from build123d import *

# Parameters (mm, degrees)
SKETCH1_W                  = 650
SKETCH1_H                  = 400
BOSS_EXTRUDE1_DEPTH        = 12
FILLET1_R                  = 10
SKETCH31_R                 = 8.15
CUT_EXTRUDE3_DEPTH         = 764.311207831
LPATTERN1_COUNT            = 9
LPATTERN1_PITCH            = 50
LPATTERN2_COUNT            = 4
LPATTERN2_PITCH            = 50
LPATTERN2_COPY_1_SKETCH_R  = 8.15
LPATTERN2_COPY_1_DEPTH     = 764.311207831
LPATTERN2_COPY_2_SKETCH_R  = 8.15
LPATTERN2_COPY_2_DEPTH     = 764.311207831
LPATTERN2_COPY_3_SKETCH_R  = 8.15
LPATTERN2_COPY_3_DEPTH     = 764.311207831
LPATTERN2_COPY_4_SKETCH_R  = 8.15
LPATTERN2_COPY_4_DEPTH     = 764.311207831
LPATTERN2_COPY_5_SKETCH_R  = 8.15
LPATTERN2_COPY_5_DEPTH     = 764.311207831
LPATTERN2_COPY_6_SKETCH_R  = 8.15
LPATTERN2_COPY_6_DEPTH     = 764.311207831
LPATTERN2_COPY_7_SKETCH_R  = 8.15
LPATTERN2_COPY_7_DEPTH     = 764.311207831
LPATTERN2_COPY_8_SKETCH_R  = 8.15
LPATTERN2_COPY_8_DEPTH     = 764.311207831
LPATTERN2_COPY_9_SKETCH_R  = 8.15
LPATTERN2_COPY_9_DEPTH     = 764.311207831
LPATTERN2_COPY_10_SKETCH_R = 8.15
LPATTERN2_COPY_10_DEPTH    = 764.311207831
LPATTERN2_COPY_11_SKETCH_R = 8.15
LPATTERN2_COPY_11_DEPTH    = 764.311207831
LPATTERN2_COPY_12_SKETCH_R = 8.15
LPATTERN2_COPY_12_DEPTH    = 764.311207831
LPATTERN2_COPY_13_SKETCH_R = 8.15
LPATTERN2_COPY_13_DEPTH    = 764.311207831
LPATTERN2_COPY_14_SKETCH_R = 8.15
LPATTERN2_COPY_14_DEPTH    = 764.311207831
LPATTERN2_COPY_15_SKETCH_R = 8.15
LPATTERN2_COPY_15_DEPTH    = 764.311207831
LPATTERN2_COPY_16_SKETCH_R = 8.15
LPATTERN2_COPY_16_DEPTH    = 764.311207831
LPATTERN2_COPY_17_SKETCH_R = 8.15
LPATTERN2_COPY_17_DEPTH    = 764.311207831
LPATTERN2_COPY_18_SKETCH_R = 8.15
LPATTERN2_COPY_18_DEPTH    = 764.311207831
LPATTERN2_COPY_19_SKETCH_R = 8.15
LPATTERN2_COPY_19_DEPTH    = 764.311207831
LPATTERN2_COPY_20_SKETCH_R = 8.15
LPATTERN2_COPY_20_DEPTH    = 764.311207831
LPATTERN2_COPY_21_SKETCH_R = 8.15
LPATTERN2_COPY_21_DEPTH    = 764.311207831
LPATTERN2_COPY_22_SKETCH_R = 8.15
LPATTERN2_COPY_22_DEPTH    = 764.311207831
LPATTERN2_COPY_23_SKETCH_R = 8.15
LPATTERN2_COPY_23_DEPTH    = 764.311207831
LPATTERN2_COPY_24_SKETCH_R = 8.15
LPATTERN2_COPY_24_DEPTH    = 764.311207831
M8_CLEARANCE_HOLE2_D       = 8.4
LPATTERN3_COUNT            = 2
LPATTERN3_PITCH            = 250
LPATTERN3_COUNT_DIR2       = 2
LPATTERN3_PITCH_DIR2       = 600


with BuildPart() as part:
    # Sketch1 → Boss-Extrude1 (new body)
    with BuildSketch(Plane(origin=(0, 0, 0), x_dir=(1, 0, 0), z_dir=(0, 1, 0))):
        with Locations((325, -200)):
            Rectangle(SKETCH1_W, SKETCH1_H)
    extrude(amount=BOSS_EXTRUDE1_DEPTH)

    # Fillet1
    fillet1_edges = [part.edges().sort_by_distance(p)[0] for p in [
        (0, 6, 0),
        (650, 6, 0),
        (650, 6, 400),
        (0, 6, 400),
    ]]
    fillet(fillet1_edges, radius=FILLET1_R)

    # Sketch31 → Cut-Extrude3 (cut, through all)
    with BuildSketch(Plane(origin=(0, 12, 0), x_dir=(1, 0, 0), z_dir=(0, 1, 0))):
        with Locations(Location((125, -275, 0), (0, 0, 270))):
            Circle(SKETCH31_R)
    cut_extrude3 = extrude(amount=-CUT_EXTRUDE3_DEPTH, mode=Mode.SUBTRACT)

    # LPattern1: Cut-Extrude3 ×9
    with Locations(*[(i * LPATTERN1_PITCH, 0, 0) for i in range(1, LPATTERN1_COUNT)]):
        add(cut_extrude3, mode=Mode.SUBTRACT)

    # LPattern2: Cut-Extrude3 ×4
    with Locations(*[(0, 0, -i * LPATTERN2_PITCH) for i in range(1, LPATTERN2_COUNT)]):
        add(cut_extrude3, mode=Mode.SUBTRACT)

    # LPattern2 copy 1 sketch → LPattern2 copy 1 (cut, through all)
    with BuildSketch(Plane(origin=(50, 12, -50), x_dir=(1, 0, 0), z_dir=(0, 1, 0))):
        with Locations(Location((125, -275, 0), (0, 0, 270))):
            Circle(LPATTERN2_COPY_1_SKETCH_R)
    extrude(amount=-LPATTERN2_COPY_1_DEPTH, mode=Mode.SUBTRACT)

    # LPattern2 copy 2 sketch → LPattern2 copy 2 (cut, through all)
    with BuildSketch(Plane(origin=(50, 12, -100), x_dir=(1, 0, 0), z_dir=(0, 1, 0))):
        with Locations(Location((125, -275, 0), (0, 0, 270))):
            Circle(LPATTERN2_COPY_2_SKETCH_R)
    extrude(amount=-LPATTERN2_COPY_2_DEPTH, mode=Mode.SUBTRACT)

    # LPattern2 copy 3 sketch → LPattern2 copy 3 (cut, through all)
    with BuildSketch(Plane(origin=(50, 12, -150), x_dir=(1, 0, 0), z_dir=(0, 1, 0))):
        with Locations(Location((125, -275, 0), (0, 0, 270))):
            Circle(LPATTERN2_COPY_3_SKETCH_R)
    extrude(amount=-LPATTERN2_COPY_3_DEPTH, mode=Mode.SUBTRACT)

    # LPattern2 copy 4 sketch → LPattern2 copy 4 (cut, through all)
    with BuildSketch(Plane(origin=(100, 12, -50), x_dir=(1, 0, 0), z_dir=(0, 1, 0))):
        with Locations(Location((125, -275, 0), (0, 0, 270))):
            Circle(LPATTERN2_COPY_4_SKETCH_R)
    extrude(amount=-LPATTERN2_COPY_4_DEPTH, mode=Mode.SUBTRACT)

    # LPattern2 copy 5 sketch → LPattern2 copy 5 (cut, through all)
    with BuildSketch(Plane(origin=(100, 12, -100), x_dir=(1, 0, 0), z_dir=(0, 1, 0))):
        with Locations(Location((125, -275, 0), (0, 0, 270))):
            Circle(LPATTERN2_COPY_5_SKETCH_R)
    extrude(amount=-LPATTERN2_COPY_5_DEPTH, mode=Mode.SUBTRACT)

    # LPattern2 copy 6 sketch → LPattern2 copy 6 (cut, through all)
    with BuildSketch(Plane(origin=(100, 12, -150), x_dir=(1, 0, 0), z_dir=(0, 1, 0))):
        with Locations(Location((125, -275, 0), (0, 0, 270))):
            Circle(LPATTERN2_COPY_6_SKETCH_R)
    extrude(amount=-LPATTERN2_COPY_6_DEPTH, mode=Mode.SUBTRACT)

    # LPattern2 copy 7 sketch → LPattern2 copy 7 (cut, through all)
    with BuildSketch(Plane(origin=(150, 12, -50), x_dir=(1, 0, 0), z_dir=(0, 1, 0))):
        with Locations(Location((125, -275, 0), (0, 0, 270))):
            Circle(LPATTERN2_COPY_7_SKETCH_R)
    extrude(amount=-LPATTERN2_COPY_7_DEPTH, mode=Mode.SUBTRACT)

    # LPattern2 copy 8 sketch → LPattern2 copy 8 (cut, through all)
    with BuildSketch(Plane(origin=(150, 12, -100), x_dir=(1, 0, 0), z_dir=(0, 1, 0))):
        with Locations(Location((125, -275, 0), (0, 0, 270))):
            Circle(LPATTERN2_COPY_8_SKETCH_R)
    extrude(amount=-LPATTERN2_COPY_8_DEPTH, mode=Mode.SUBTRACT)

    # LPattern2 copy 9 sketch → LPattern2 copy 9 (cut, through all)
    with BuildSketch(Plane(origin=(150, 12, -150), x_dir=(1, 0, 0), z_dir=(0, 1, 0))):
        with Locations(Location((125, -275, 0), (0, 0, 270))):
            Circle(LPATTERN2_COPY_9_SKETCH_R)
    extrude(amount=-LPATTERN2_COPY_9_DEPTH, mode=Mode.SUBTRACT)

    # LPattern2 copy 10 sketch → LPattern2 copy 10 (cut, through all)
    with BuildSketch(Plane(origin=(200, 12, -50), x_dir=(1, 0, 0), z_dir=(0, 1, 0))):
        with Locations(Location((125, -275, 0), (0, 0, 270))):
            Circle(LPATTERN2_COPY_10_SKETCH_R)
    extrude(amount=-LPATTERN2_COPY_10_DEPTH, mode=Mode.SUBTRACT)

    # LPattern2 copy 11 sketch → LPattern2 copy 11 (cut, through all)
    with BuildSketch(Plane(origin=(200, 12, -100), x_dir=(1, 0, 0), z_dir=(0, 1, 0))):
        with Locations(Location((125, -275, 0), (0, 0, 270))):
            Circle(LPATTERN2_COPY_11_SKETCH_R)
    extrude(amount=-LPATTERN2_COPY_11_DEPTH, mode=Mode.SUBTRACT)

    # LPattern2 copy 12 sketch → LPattern2 copy 12 (cut, through all)
    with BuildSketch(Plane(origin=(200, 12, -150), x_dir=(1, 0, 0), z_dir=(0, 1, 0))):
        with Locations(Location((125, -275, 0), (0, 0, 270))):
            Circle(LPATTERN2_COPY_12_SKETCH_R)
    extrude(amount=-LPATTERN2_COPY_12_DEPTH, mode=Mode.SUBTRACT)

    # LPattern2 copy 13 sketch → LPattern2 copy 13 (cut, through all)
    with BuildSketch(Plane(origin=(250, 12, -50), x_dir=(1, 0, 0), z_dir=(0, 1, 0))):
        with Locations(Location((125, -275, 0), (0, 0, 270))):
            Circle(LPATTERN2_COPY_13_SKETCH_R)
    extrude(amount=-LPATTERN2_COPY_13_DEPTH, mode=Mode.SUBTRACT)

    # LPattern2 copy 14 sketch → LPattern2 copy 14 (cut, through all)
    with BuildSketch(Plane(origin=(250, 12, -100), x_dir=(1, 0, 0), z_dir=(0, 1, 0))):
        with Locations(Location((125, -275, 0), (0, 0, 270))):
            Circle(LPATTERN2_COPY_14_SKETCH_R)
    extrude(amount=-LPATTERN2_COPY_14_DEPTH, mode=Mode.SUBTRACT)

    # LPattern2 copy 15 sketch → LPattern2 copy 15 (cut, through all)
    with BuildSketch(Plane(origin=(250, 12, -150), x_dir=(1, 0, 0), z_dir=(0, 1, 0))):
        with Locations(Location((125, -275, 0), (0, 0, 270))):
            Circle(LPATTERN2_COPY_15_SKETCH_R)
    extrude(amount=-LPATTERN2_COPY_15_DEPTH, mode=Mode.SUBTRACT)

    # LPattern2 copy 16 sketch → LPattern2 copy 16 (cut, through all)
    with BuildSketch(Plane(origin=(300, 12, -50), x_dir=(1, 0, 0), z_dir=(0, 1, 0))):
        with Locations(Location((125, -275, 0), (0, 0, 270))):
            Circle(LPATTERN2_COPY_16_SKETCH_R)
    extrude(amount=-LPATTERN2_COPY_16_DEPTH, mode=Mode.SUBTRACT)

    # LPattern2 copy 17 sketch → LPattern2 copy 17 (cut, through all)
    with BuildSketch(Plane(origin=(300, 12, -100), x_dir=(1, 0, 0), z_dir=(0, 1, 0))):
        with Locations(Location((125, -275, 0), (0, 0, 270))):
            Circle(LPATTERN2_COPY_17_SKETCH_R)
    extrude(amount=-LPATTERN2_COPY_17_DEPTH, mode=Mode.SUBTRACT)

    # LPattern2 copy 18 sketch → LPattern2 copy 18 (cut, through all)
    with BuildSketch(Plane(origin=(300, 12, -150), x_dir=(1, 0, 0), z_dir=(0, 1, 0))):
        with Locations(Location((125, -275, 0), (0, 0, 270))):
            Circle(LPATTERN2_COPY_18_SKETCH_R)
    extrude(amount=-LPATTERN2_COPY_18_DEPTH, mode=Mode.SUBTRACT)

    # LPattern2 copy 19 sketch → LPattern2 copy 19 (cut, through all)
    with BuildSketch(Plane(origin=(350, 12, -50), x_dir=(1, 0, 0), z_dir=(0, 1, 0))):
        with Locations(Location((125, -275, 0), (0, 0, 270))):
            Circle(LPATTERN2_COPY_19_SKETCH_R)
    extrude(amount=-LPATTERN2_COPY_19_DEPTH, mode=Mode.SUBTRACT)

    # LPattern2 copy 20 sketch → LPattern2 copy 20 (cut, through all)
    with BuildSketch(Plane(origin=(350, 12, -100), x_dir=(1, 0, 0), z_dir=(0, 1, 0))):
        with Locations(Location((125, -275, 0), (0, 0, 270))):
            Circle(LPATTERN2_COPY_20_SKETCH_R)
    extrude(amount=-LPATTERN2_COPY_20_DEPTH, mode=Mode.SUBTRACT)

    # LPattern2 copy 21 sketch → LPattern2 copy 21 (cut, through all)
    with BuildSketch(Plane(origin=(350, 12, -150), x_dir=(1, 0, 0), z_dir=(0, 1, 0))):
        with Locations(Location((125, -275, 0), (0, 0, 270))):
            Circle(LPATTERN2_COPY_21_SKETCH_R)
    extrude(amount=-LPATTERN2_COPY_21_DEPTH, mode=Mode.SUBTRACT)

    # LPattern2 copy 22 sketch → LPattern2 copy 22 (cut, through all)
    with BuildSketch(Plane(origin=(400, 12, -50), x_dir=(1, 0, 0), z_dir=(0, 1, 0))):
        with Locations(Location((125, -275, 0), (0, 0, 270))):
            Circle(LPATTERN2_COPY_22_SKETCH_R)
    extrude(amount=-LPATTERN2_COPY_22_DEPTH, mode=Mode.SUBTRACT)

    # LPattern2 copy 23 sketch → LPattern2 copy 23 (cut, through all)
    with BuildSketch(Plane(origin=(400, 12, -100), x_dir=(1, 0, 0), z_dir=(0, 1, 0))):
        with Locations(Location((125, -275, 0), (0, 0, 270))):
            Circle(LPATTERN2_COPY_23_SKETCH_R)
    extrude(amount=-LPATTERN2_COPY_23_DEPTH, mode=Mode.SUBTRACT)

    # LPattern2 copy 24 sketch → LPattern2 copy 24 (cut, through all)
    with BuildSketch(Plane(origin=(400, 12, -150), x_dir=(1, 0, 0), z_dir=(0, 1, 0))):
        with Locations(Location((125, -275, 0), (0, 0, 270))):
            Circle(LPATTERN2_COPY_24_SKETCH_R)
    extrude(amount=-LPATTERN2_COPY_24_DEPTH, mode=Mode.SUBTRACT)

    # M8 Clearance Hole2 (through all)
    with Locations(Plane(origin=(0, 0, 0), x_dir=(-1, 0, 0), z_dir=(0, -1, 0))):
        with Locations((-25, -75)):
            m8_clearance_hole2 = Hole(M8_CLEARANCE_HOLE2_D / 2)

    # LPattern3: M8 Clearance Hole2 2 × 2
    with Locations(*[(j * LPATTERN3_PITCH_DIR2, 0, i * LPATTERN3_PITCH) for i in range(LPATTERN3_COUNT) for j in range(LPATTERN3_COUNT_DIR2) if (i, j) != (0, 0)]):
        add(m8_clearance_hole2, mode=Mode.SUBTRACT)


solid = part.part
The listing builds one solid part. Answer for the finished solid, in the listing's coordinates (mm). Coordinates: 2 decimals unless noted, no trailing zeros. Write each loop counter-clockwise with the first axis right and the second up, starting at its lowest first coordinate (ties: lowest second). Pieces come first, ordered by that corner, then holes. Notation, with made-up numbers: (-4.5, -3) - (7.5, -3) arc R24 ccw to (7.5, 18) - close; hole circle Ø1 at (60.25, 79.25). An arc over 180 degrees is marked (long way). Put each result on its own line as item: value.
1. The part is cut by section A-A on x = 425. Give the vertices of the cut face in (y, z).
Answer sheet:
outline: (0, 0) - (12, 0) - (12, 116.85) - (0, 116.85) - close; (0, 133.15) - (12, 133.15) - (12, 166.85) - (0, 166.85) - close; (0, 183.15) - (12, 183.15) - (12, 216.85) - (0, 216.85) - close; (0, 233.15) - (12, 233.15) - (12, 266.85) - (0, 266.85) - close; (0, 283.15) - (12, 283.15) - (12, 400) - (0, 400) - close
2. The part is cut by section B-B on y = 2.5. State how many separate pieces and enclosed holes the cut face has, plus the area to 3 significant figures.
Answer sheet:
separate pieces: 1
enclosed holes: 40
area: 252,000 mm^2
3. Find the intervals of material crossed by line 1 along Z through (x, y) = (520.5, 6.25); line 2 along X through (y, z) = (4, 77); line 3 along Z through (x, y) = (182, 7), in increasing order. Write a range as from..to.
Answer sheet:
line 1: z = 0..118.2, 131.8..168.2, 181.8..218.2, 231.8..268.2, 281.8..400
line 2: x = 0..21.31, 28.69..621.31, 628.69..650
line 3: z = 0..120.83, 129.17..170.83, 179.17..220.83, 229.17..270.83, 279.17..400
4. Determine the mould class of faces 1 (the face through (220.041, 6.084, 268.532)), 2 (the face through (320, 12, 197)) for opening direction Z: pulls with the +Z half, pulls with the -Z half, needs draft (parallel to the pull), parting line crosses it, or undercut.
Answer sheet:
face 1: undercut
face 2: needs draft
5. A flat-ended cylindrical pin translates along its axis: pin 1 Ø14.5 at (x, z) = (525, 275) entering from -Y. Find the tip coordinate at first contact, or state that the pin passes through.
Answer sheet:
pin 1: passes through
